```python
from build123d import *

# Parameters (mm, degrees)
SKETCH_1_R          = 50
SKETCH_1_R_2        = 2
EXTRUDE_1_DEPTH     = 10
SKETCH_2_R          = 22
SKETCH_2_R_2        = 10
CUT_EXTRUDE_1_DEPTH = 5
SKETCH_2_3_R        = 1.75
SKETCH_2_3_R_2      = 10
CUT_EXTRUDE_2_DEPTH = 75.1479844


with BuildPart() as part:
    # Sketch 1 → Extrude 1 (new body)
    # profile 1 of 5: a face of its own
    with BuildSketch(Plane(origin=(0, 0, 0), x_dir=(1, 0, 0), z_dir=(0, 1, 0))):
        Circle(SKETCH_1_R)
        with BuildLine():
            ThreePointArc((-28.838834765, 32.374368671), (-32.374368671, 32.374368671), (-32.374368671, 28.838834765))
            Line((-32.374368671, 28.838834765), (-21.767766953, 18.232233047))
            ThreePointArc((-21.767766953, 18.232233047), (-18.232233047, 18.232233047), (-18.232233047, 21.767766953))
            Line((-18.232233047, 21.767766953), (-28.838834765, 32.374368671))
        make_face(mode=Mode.SUBTRACT)
        with BuildLine():
            ThreePointArc((-32.374368671, -28.838834765), (-32.374368671, -32.374368671), (-28.838834765, -32.374368671))
            Line((-28.838834765, -32.374368671), (-18.232233047, -21.767766953))
            ThreePointArc((-18.232233047, -21.767766953), (-18.232233047, -18.232233047), (-21.767766953, -18.232233047))
            Line((-21.767766953, -18.232233047), (-32.374368671, -28.838834765))
        make_face(mode=Mode.SUBTRACT)
        with BuildLine():
            ThreePointArc((28.838834765, -32.374368671), (32.374368671, -32.374368671), (32.374368671, -28.838834765))
            Line((32.374368671, -28.838834765), (21.767766953, -18.232233047))
            ThreePointArc((21.767766953, -18.232233047), (18.232233047, -18.232233047), (18.232233047, -21.767766953))
            Line((18.232233047, -21.767766953), (28.838834765, -32.374368671))
        make_face(mode=Mode.SUBTRACT)
        with BuildLine():
            ThreePointArc((32.374368671, 28.838834765), (32.374368671, 32.374368671), (28.838834765, 32.374368671))
            Line((28.838834765, 32.374368671), (18.232233047, 21.767766953))
            ThreePointArc((18.232233047, 21.767766953), (18.232233047, 18.232233047), (21.767766953, 18.232233047))
            Line((21.767766953, 18.232233047), (32.374368671, 28.838834765))
        make_face(mode=Mode.SUBTRACT)
    # profile 2 of 5: a face of its own
    with BuildSketch(Plane(origin=(0, 0, 0), x_dir=(1, 0, 0), z_dir=(0, 1, 0))):
        with BuildLine():
            ThreePointArc((-31.466251763, -48.436814511), (-25.799706685, -45.41900176), (-19.413503243, -46.077281732))
            ThreePointArc((-19.413503243, -46.077281732), (-35.355339059, -35.355339059), (-46.077281732, -19.413503243))
            ThreePointArc((-46.077281732, -19.413503243), (-45.41900176, -25.799706685), (-48.436814511, -31.466251763))
            ThreePointArc((-48.436814511, -31.466251763), (-48.436814511, -48.436814511), (-31.466251763, -48.436814511))
        make_face()
        with Locations(Location((-39.951533137, -39.951533137, 0), (0, 0, 270))):
            Circle(SKETCH_1_R_2, mode=Mode.SUBTRACT)
    # profile 3 of 5: a face of its own
    with BuildSketch(Plane(origin=(0, 0, 0), x_dir=(1, 0, 0), z_dir=(0, 1, 0))):
        with BuildLine():
            ThreePointArc((48.436814511, -31.466251763), (45.41900176, -25.799706685), (46.077281732, -19.413503243))
            ThreePointArc((46.077281732, -19.413503243), (35.355339059, -35.355339059), (19.413503243, -46.077281732))
            ThreePointArc((19.413503243, -46.077281732), (25.799706685, -45.41900176), (31.466251763, -48.436814511))
            ThreePointArc((31.466251763, -48.436814511), (48.436814511, -48.436814511), (48.436814511, -31.466251763))
        make_face()
        with Locations(Location((39.951533137, -39.951533137, 0), (0, 0, 270))):
            Circle(SKETCH_1_R_2, mode=Mode.SUBTRACT)
    # profile 4 of 5: a face of its own
    with BuildSketch(Plane(origin=(0, 0, 0), x_dir=(1, 0, 0), z_dir=(0, 1, 0))):
        with BuildLine():
            ThreePointArc((19.413503243, 46.077281732), (35.355339059, 35.355339059), (46.077281732, 19.413503243))
            ThreePointArc((46.077281732, 19.413503243), (45.41900176, 25.799706685), (48.436814511, 31.466251763))
            ThreePointArc((48.436814511, 31.466251763), (48.436814511, 48.436814511), (31.466251763, 48.436814511))
            ThreePointArc((31.466251763, 48.436814511), (25.799706685, 45.41900176), (19.413503243, 46.077281732))
        make_face()
        with Locations(Location((39.951533137, 39.951533137, 0), (0, 0, 270))):
            Circle(SKETCH_1_R_2, mode=Mode.SUBTRACT)
    # profile 5 of 5: a face of its own
    with BuildSketch(Plane(origin=(0, 0, 0), x_dir=(1, 0, 0), z_dir=(0, 1, 0))):
        with BuildLine():
            ThreePointArc((-46.077281732, 19.413503243), (-35.355339059, 35.355339059), (-19.413503243, 46.077281732))
            ThreePointArc((-19.413503243, 46.077281732), (-25.799706685, 45.41900176), (-31.466251763, 48.436814511))
            ThreePointArc((-31.466251763, 48.436814511), (-48.436814511, 48.436814511), (-48.436814511, 31.466251763))
            ThreePointArc((-48.436814511, 31.466251763), (-45.41900176, 25.799706685), (-46.077281732, 19.413503243))
        make_face()
        with Locations(Location((-39.951533137, 39.951533137, 0), (0, 0, 270))):
            Circle(SKETCH_1_R_2, mode=Mode.SUBTRACT)
    extrude(amount=EXTRUDE_1_DEPTH)

    # Sketch 2 → Cut-Extrude 1 (cut)
    with BuildSketch(Plane(origin=(0, 10, 0), x_dir=(1, 0, 0), z_dir=(0, 1, 0))):
        with Locations(Location((0, 0, 0), (0, 0, 270))):
            Circle(SKETCH_2_R)
        with Locations(Location((0, 0, 0), (0, 0, 270))):
            Circle(SKETCH_2_R_2, mode=Mode.SUBTRACT)
    extrude(amount=-CUT_EXTRUDE_1_DEPTH, mode=Mode.SUBTRACT)

    # Sketch 2_3 → Cut-Extrude 2 (cut, through all)
    with BuildSketch(Plane(origin=(0, 10, 0), x_dir=(1, 0, 0), z_dir=(0, 1, 0))):
        with Locations(Location((-12.557368355, -7.25, 0), (0, 0, 270))):
            Circle(SKETCH_2_3_R)
        with Locations(Location((12.557368355, -7.25, 0), (0, 0, 270))):
            Circle(SKETCH_2_3_R)
        with Locations(Location((0, 14.5, 0), (0, 0, 270))):
            Circle(SKETCH_2_3_R)
        with Locations(Location((0, 0, 0), (0, 0, 270))):
            Circle(SKETCH_2_3_R_2)
    extrude(amount=-CUT_EXTRUDE_2_DEPTH, mode=Mode.SUBTRACT)


solid = part.part
```
Check sheet for the modelled part. Datum: model origin and axes. Units: mm. A direction names the side the tool comes from. Round coordinates to 2 decimals unless told otherwise and drop trailing zeros. Loops run counter-clockwise (first coordinate to the right, second up) from the corner with the lowest first, then second, coordinate; pieces in that order, holes last. Notation, with made-up numbers: (-1, 72.25) -> (20, 72.25) arc R24 ccw to (20, 88.25) -> close; hole circle Ø3 at (-26.5, -14). An arc over 180 degrees is marked (long way). Answer in a Markdown table with one row per item.
Q1. Sectioned sample at C-C on z = -40. Enter the section's corners in (x, y), then the cut area to 3 significant figures.
Data:
| item | result |
|---|---|
| outline | (-51.95, 0) -> (-41.95, 0) -> (-41.95, 10) -> (-51.95, 10) -> close; (-37.95, 0) -> (37.95, 0) -> (37.95, 10) -> (-37.95, 10) -> close; (41.95, 0) -> (51.95, 0) -> (51.95, 10) -> (41.95, 10) -> close |
| area | 959 mm^2 |
Q2. Thickness scan on L1, parallel to Z at x = 19, y = 5.25; L2, parallel to X at y = 3.25, z = 19.5; L3, parallel to Z at x = 40, y = 0.5. Record the ranges inside material, lowest first.
Data:
| item | result |
|---|---|
| L1 | z = -46.25 to -22.54, -17.71 to -11.09, 11.09 to 17.71, 22.54 to 46.25 |
| L2 | x = -46.04 to -23.04, -17.55 to 17.55, 23.04 to 46.04 |
| L3 | z = -51.95 to -41.95, -37.95 to 37.95, 41.95 to 51.95 |
Q3. Go/stop test with flat-tipped pins: P1, Ø2, axis at x = -3.5, y = 4.5, coming from the -Z side; P2, Ø3, axis at x = -30.5, y = 4.5, coming from the -Z side; P3, Ø5, axis at x = -21, y = 8.5, coming from the +Z side. Record where each tip stops, or that it passes through.
Data:
| item | result |
|---|---|
| P1 | stops at z = -49.94 |
| P2 | stops at z = -48.94 |
| P3 | stops at z = 46.45 |
Q4. Set-up check for faces 1 (the face through (23.461, 4.93, 26.997)), 2 (the face through (0, 5, -50)): record each of +Z, -Z, +X, -X, +Y, -Y from which the full face is reachable in a straight line by a thin tool's end or side.
Data:
| item | result |
|---|---|
| face 1 | +Y, -Y |
| face 2 | -Z, +Y, -Y |
Q5. Sectioned sample at D-D on y = 2.25. Give the number of separate pieces and of enclosed holes in the cut face, then the cut area to 3 significant figures.
Data:
| item | result |
|---|---|
| separate pieces | 1 |
| enclosed holes | 12 |
| area | 8,750 mm^2 |
Q6. Sectioned sample at A-A on z = 0. Enter the section's corners in (x, y).
Data:
| item | result |
|---|---|
| outline | (-50, 0) -> (-10, 0) -> (-10, 5) -> (-22, 5) -> (-22, 10) -> (-50, 10) -> close; (10, 0) -> (50, 0) -> (50, 10) -> (22, 10) -> (22, 5) -> (10, 5) -> close |
Q7. Sectioned sample at B-B on x = 0. Enter the section's corners in (y, z).
Data:
| item | result |
|---|---|
| outline | (0, -50) -> (10, -50) -> (10, -22) -> (5, -22) -> (5, -16.25) -> (0, -16.25) -> close; (0, -12.75) -> (5, -12.75) -> (5, -10) -> (0, -10) -> close; (0, 10) -> (5, 10) -> (5, 22) -> (10, 22) -> (10, 50) -> (0, 50) -> close |
